```python
from build123d import *

# Parameters (mm, degrees)
BOSS_EXTRUDE1_DEPTH = 174.625
FILLET1_R           = 1.016


with BuildPart() as part:
    # Sketch1 → Boss-Extrude1 (new body)
    with BuildSketch(Plane.XY):
        with BuildLine():
            Line((0, 11.90625), (0, 18.25625))
            Line((0, 18.25625), (-4.7625, 18.25625))
            Line((-4.7625, 18.25625), (-4.7625, 13.4575956))
            ThreePointArc((-4.7625, 13.4575956), (-7.045294516, 7.570988051), (-12.7, 4.7625))
            Line((-12.7, 4.7625), (-12.7, 0))
            Line((-12.7, 0), (-3.476318041, 0))
            Line((-3.476318041, 0), (-1.738159021, 1.738159021))
            Line((-1.738159021, 1.738159021), (-0.79375, 0.79375))
            Line((-0.79375, 0.79375), (-0.07532951, 1.51217049))
            Line((-0.07532951, 1.51217049), (-1.738159021, 3.175))
            Line((-1.738159021, 3.175), (-3.897159021, 1.016))
            Line((-3.897159021, 1.016), (-11.684, 1.016))
            Line((-11.684, 1.016), (-11.684, 3.879825113))
            ThreePointArc((-11.684, 3.879825113), (-5.988786034, 7.237917278), (-3.7465, 13.4575956))
            Line((-3.7465, 13.4575956), (-3.7465, 17.24025))
            Line((-3.7465, 17.24025), (-1.016, 17.24025))
            Line((-1.016, 17.24025), (-1.016, 11.90625))
            Line((-1.016, 11.90625), (0, 11.90625))
        make_face()
    extrude(amount=-BOSS_EXTRUDE1_DEPTH)

    # Fillet1
    fillet1_edges = [part.edges().sort_by_distance(p)[0] for p in [
        (-1.738159021, 3.175, -87.3125),
        (-3.476318041, 0, -87.3125),
        (-12.7, 0, -87.3125),
        (-12.7, 4.7625, -87.3125),
        (-4.7625, 18.25625, -87.3125),
        (0, 18.25625, -87.3125),
    ]]
    fillet(fillet1_edges, radius=FILLET1_R)


solid = part.part
```
Geometry check sheet. Reference: the model listing, model coordinates, mm. A direction names the side the tool comes from. Give positions to 0.01 mm unless a question says otherwise; leave off trailing zeros. Order: outer loops, then holes, each group sorted by start corner. A loop starts at its lowest first (then second) coordinate and runs counter-clockwise, first axis right, second up. Notation, with made-up numbers: (27, 67.25) -> (58, 67.25) arc R18 ccw to (58, 72.25) -> close; hole circle Ø11 at (-7.5, 44.5). An arc over 180 degrees is marked (long way). Write each question's results on one line, items separated by ' | '. Start each with the question number.
(1) Mould release check, pull along X, two halves, no side actions. Record for faces 1 (the face through (-6.72, 7.95, -86.09)), 2 (the face through (-11.684, 2, -86)), 3 (the face through (-5.4, 8.5, -174.625)), 4 (the face through (-2, 17.24, -86)): pulls with the +X half, pulls with the -X half, needs draft (parallel to the pull), parting line crosses it, or undercut.
(2) Scan lines: line 1 (X direction, y = 15.75, z = -143); line 2 (Y direction, x = -9.5, z = -17); line 3 (X direction, y = 2.5, z = -52). Record each from-to range of solid material in increasing order.
(3) Sectioned sample at B-B (x = -9.5). Enter the section's corners in (y, z) (3 decimals).
(4) Gauge pin test, flat ends, axial feed: P1, Ø4.5, axis at y = 14, z = -107.5, coming from the -X side; P2, Ø1.4, axis at y = 2, z = -90.5, coming from the +X side; P3, Ø6, axis at x = -9.5, z = -107, coming from the +Y side. Record the tip position at first contact, or that the pin passes through.
(5) Access from +Z, -Z, +X, -X, +Y, -Y to the whole of each face (thin tool, end or side, straight path). Record for faces 5 (the face through (-5.4, 8.5, 0)), 6 (the face through (-4.762, 15, -86)), 7 (the face through (-1.016, 15, -86)).
(6) Sectioned sample at C-C (y = 6.5). Enter the section's corners in (x, z) (3 decimals).
(7) Sectioned sample at A-A (z = -131.5). Enter the section's corners in (x, y), plus the area to 3 significant figures.
Answer below:
1) face 1: pulls with the -X half | face 2: undercut | face 3: needs draft | face 4: undercut
2) line 1: -4.76 to -3.75, -1.02 to 0 | line 2: 0 to 1.02, 4.57 to 5.69 | line 3: -12.7 to -11.68, -2.41 to -1.07
3) outline: (0, -174.625) -> (1.016, -174.625) -> (1.016, 0) -> (0, 0) -> close; (4.566, -174.625) -> (5.693, -174.625) -> (5.693, 0) -> (4.566, 0) -> close
4) P1: x = -4.93 | P2: x = -0.08 | P3: y = 8.23
5) face 5: +Z, +X, -X, +Y, -Y | face 6: +Z, -Z, -X, +Y | face 7: +Z, -Z
6) outline: (-8.219, -174.625) -> (-6.667, -174.625) -> (-6.667, 0) -> (-8.219, 0) -> close
7) outline: (-12.7, 1.02) arc R1.02 ccw to (-11.68, 0) -> (-3.9, 0) arc R1.02 ccw to (-3.18, 0.3) -> (-1.74, 1.74) -> (-0.79, 0.79) -> (-0.08, 1.51) -> (-1.02, 2.46) arc R1.02 ccw to (-2.46, 2.46) -> (-3.9, 1.02) -> (-11.68, 1.02) -> (-11.68, 3.88) arc R9.75 ccw to (-3.75, 13.46) -> (-3.75, 17.24) -> (-1.02, 17.24) -> (-1.02, 11.91) -> (0, 11.91) -> (0, 17.24) arc R1.02 ccw to (-1.02, 18.26) -> (-3.75, 18.26) arc R1.02 ccw to (-4.76, 17.24) -> (-4.76, 13.46) arc R8.73 cw to (-11.87, 4.88) arc R1.02 ccw to (-12.7, 3.88) -> close | area: 43.6 mm2
